from build123d import *

# Parameters (mm, degrees)
F0_W     = 300
F0_H     = 15
F1_DEPTH = 3
F2_DEPTH = 6
F3_R     = 1.25
F3_W     = 2
F3_H     = 12
F5_DEPTH = 2
F4_W     = 2
F4_H     = 12
F4_R     = 1.25
F6_DEPTH = 2


with BuildPart() as f1:
    # F0 (on Front) → F1 (new body)
    with BuildSketch(Plane.XZ):
        Rectangle(F0_W, F0_H)
    extrude(amount=F1_DEPTH)

    # F0 (on Front) → F2 (join)
    with BuildSketch(Plane.XZ):
        Rectangle(F0_W, F0_H)
    extrude(amount=-F2_DEPTH)

    # F3 (on face) → F5 (join)
    with BuildSketch(Plane.XZ.offset(3)):
        with BuildLine():
            ThreePointArc((-156.25, 0), (-157.48712, 2.296452), (-160.085414, 2.526733))
            ThreePointArc((-160.085414, 2.526733), (-161.75, 0), (-160.085414, -2.526733))
            ThreePointArc((-160.085414, -2.526733), (-157.48712, -2.296452), (-156.25, 0))
        make_face()
        with Locations((-159, 0)):
            Circle(F3_R, mode=Mode.SUBTRACT)
        with BuildLine():
            Line((-152, -6), (-152, 6))
            Line((-152, 6), (-160.085414, 2.526733))
            ThreePointArc((-160.085414, 2.526733), (-157.48712, 2.296452), (-156.25, 0))
            ThreePointArc((-156.25, 0), (-157.48712, -2.296452), (-160.085414, -2.526733))
            Line((-160.085414, -2.526733), (-152, -6))
        make_face()
        with Locations((-151, 0)):
            Rectangle(F3_W, F3_H)
        with Locations((151, 0)):
            Rectangle(F3_W, F3_H)
        with BuildLine():
            ThreePointArc((160.085414, -2.526733), (156.25, 0), (160.085414, 2.526733))
            Line((160.085414, 2.526733), (152, 6))
            Line((152, 6), (152, -6))
            Line((152, -6), (160.085414, -2.526733))
        make_face()
        with BuildLine():
            ThreePointArc((160.085414, -2.526733), (161.296452, -1.51288), (161.75, 0))
            ThreePointArc((161.75, 0), (161.296452, 1.51288), (160.085414, 2.526733))
            ThreePointArc((160.085414, 2.526733), (156.25, 0), (160.085414, -2.526733))
        make_face()
        with Locations((159, 0)):
            Circle(F3_R, mode=Mode.SUBTRACT)
    extrude(amount=-F5_DEPTH)

    # F4 (on face) → F6 (join)
    with BuildSketch(Plane(origin=(0, 6, 0), x_dir=(-1, 0, 0), z_dir=(0, 1, 0))):
        with BuildLine():
            Line((-152, -6), (-152, 6))
            Line((-152, 6), (-160.085414, 2.526733))
            ThreePointArc((-160.085414, 2.526733), (-157.48712, 2.296452), (-156.25, 0))
            ThreePointArc((-156.25, 0), (-157.48712, -2.296452), (-160.085414, -2.526733))
            Line((-160.085414, -2.526733), (-152, -6))
        make_face()
        with Locations((-151, 0)):
            Rectangle(F4_W, F4_H)
        with BuildLine():
            ThreePointArc((-156.25, 0), (-157.48712, 2.296452), (-160.085414, 2.526733))
            ThreePointArc((-160.085414, 2.526733), (-161.75, 0), (-160.085414, -2.526733))
            ThreePointArc((-160.085414, -2.526733), (-157.48712, -2.296452), (-156.25, 0))
        make_face()
        with Locations((-159, 0)):
            Circle(F4_R, mode=Mode.SUBTRACT)
        with Locations((151, 0)):
            Rectangle(F4_W, F4_H)
        with BuildLine():
            ThreePointArc((160.085414, -2.526733), (156.25, 0), (160.085414, 2.526733))
            Line((160.085414, 2.526733), (152, 6))
            Line((152, 6), (152, -6))
            Line((152, -6), (160.085414, -2.526733))
        make_face()
        with BuildLine():
            ThreePointArc((160.085414, -2.526733), (161.296452, -1.51288), (161.75, 0))
            ThreePointArc((161.75, 0), (161.296452, 1.51288), (160.085414, 2.526733))
            ThreePointArc((160.085414, 2.526733), (156.25, 0), (160.085414, -2.526733))
        make_face()
        with Locations((159, 0)):
            Circle(F4_R, mode=Mode.SUBTRACT)
    extrude(amount=-F6_DEPTH)


solid = f1.part
Can you work these out from the model? Positions are in its coordinate system, mm. A direction names the side the tool comes from. Coordinates: 2 decimals unless noted, no trailing zeros. Loops run counter-clockwise (first coordinate to the right, second up) from the corner with the lowest first, then second, coordinate; pieces in that order, holes last. Notation, with made-up numbers: M -25,46.5 L 34,46.5 A10 cw 34,65.5 Z; hole C 55.5,51.5 d6. An arc over 180 degrees is marked long. Answer as CSV lines item,"result". Start each with the question number.
1. Thinking about a two-plate mould opening in Y: for faces 1 (the face through (-2, -3, 0)), 2 (the face through (-2, 1, 7.5)), 3 (the face through (-2, 6, 0)), 4 (the face through (-154, 4, 0)), which applies, +Y half, -Y half, draft (parallel to the pull), parting line (faces both ways), or undercut?
2. For faces 5 (the face through (155, 4, 0)), 6 (the face through (-2, 1, -7.5)), 7 (the face through (-155, -1, 0)), which set-ups out of +Z, -Z, +X, -X, +Y, -Y let a thin tool reach every point of the face, with its end or its side?
3. If I drill on probe 1 along X at (y, z) = (2, -6.5); probe 2 along Z at (x, y) = (159, -1.8); probe 3 along X at (y, z) = (-1.75, 5.5), over which ranges is the centre line in solid material (lowest first)? Write a range as [from, to].
4. Suppose I cut it at A-A, the plane y = 1. List the corners of the cut face in (x, z) for me.
5. For pin 1 Ø2.5 at (y, z) = (0.5, 0.5) entering from +X; pin 2 Ø1 at (x, y) = (-151, 5) entering from -Z; pin 3 Ø1.6 at (x, y) = (-151, 5) entering from +Z, each with a flat end and sliding along its axis, tell me the tip position at first contact or that it passes through.
Output:
1,face 1,"-Y half"
1,face 2,"draft"
1,face 3,"+Y half"
1,face 4,"undercut"
2,face 5,"+Z, -Z, +X"
2,face 6,"-Z, +X, -X, +Y, -Y"
2,face 7,"+Z, -Z, -X"
3,probe 1,"x = [-150, 150]"
3,probe 2,"z = [-2.99, -1.25], [1.25, 2.99]"
3,probe 3,"x = [-153.16, 153.16]"
4,outline,"M -150,-7.5 L 150,-7.5 L 150,7.5 L -150,7.5 Z"
5,pin 1,"stops at x = 150"
5,pin 2,"stops at z = -6"
5,pin 3,"stops at z = 6"
